from build123d import *

# Parameters (mm, degrees)
SKETCH2_W           = 96
SKETCH2_H           = 48
BOSS_EXTRUDE1_DEPTH = 12.7
SKETCH1_R           = 48
SKETCH1_R_2         = 23.5
SKETCH1_R_3         = 1
BOSS_EXTRUDE2_DEPTH = 12.7
SKETCH1_2_R         = 23.5
SKETCH1_2_R_2       = 1
CUT_EXTRUDE1_DEPTH  = 12.7
SKETCH3_R           = 30
CUT_EXTRUDE3_DEPTH  = 5
CHAMFER1_SIZE       = 0.5


with BuildPart() as part:
    # Sketch2 → Boss-Extrude1 (new body)
    with BuildSketch(Plane(origin=(0, 0, 0), x_dir=(1, 0, 0), z_dir=(0, 1, 0))):
        with Locations((0, 24)):
            Rectangle(SKETCH2_W, SKETCH2_H)
    extrude(amount=BOSS_EXTRUDE1_DEPTH)

    # Sketch1 → Boss-Extrude2 (add)
    with BuildSketch(Plane(origin=(0, 0, 0), x_dir=(1, 0, 0), z_dir=(0, 1, 0))):
        Circle(SKETCH1_R)
        Circle(SKETCH1_R_2, mode=Mode.SUBTRACT)
        with Locations((0, 44)):
            Circle(SKETCH1_R_3, mode=Mode.SUBTRACT)
        with Locations((34.400585229, 27.433551282)):
            Circle(SKETCH1_R_3, mode=Mode.SUBTRACT)
        with Locations(Location((42.896828136, -9.790921094, 0), (0, 0, 270))):
            Circle(SKETCH1_R_3, mode=Mode.SUBTRACT)
        with Locations(Location((19.090884521, -39.642630188, 0), (0, 0, 270))):
            Circle(SKETCH1_R_3, mode=Mode.SUBTRACT)
        with Locations(Location((-19.090884521, -39.642630188, 0), (0, 0, 270))):
            Circle(SKETCH1_R_3, mode=Mode.SUBTRACT)
        with Locations(Location((-42.896828136, -9.790921094, 0), (0, 0, 270))):
            Circle(SKETCH1_R_3, mode=Mode.SUBTRACT)
        with Locations((-34.400585229, 27.433551282)):
            Circle(SKETCH1_R_3, mode=Mode.SUBTRACT)
    extrude(amount=BOSS_EXTRUDE2_DEPTH)

    # Sketch1_2 → Cut-Extrude1 (cut)
    with BuildSketch(Plane(origin=(0, 0, 0), x_dir=(1, 0, 0), z_dir=(0, 1, 0))):
        with Locations(Location((0, 0, 0), (0, 0, 270))):
            Circle(SKETCH1_2_R)
        with Locations(Location((0, 44, 0), (0, 0, 270))):
            Circle(SKETCH1_2_R_2)
        with Locations(Location((34.400585229, 27.433551282, 0), (0, 0, 270))):
            Circle(SKETCH1_2_R_2)
        with Locations(Location((-34.400585229, 27.433551282, 0), (0, 0, 270))):
            Circle(SKETCH1_2_R_2)
    extrude(amount=CUT_EXTRUDE1_DEPTH, mode=Mode.SUBTRACT)

    # Sketch3 → Cut-Extrude3 (cut)
    with BuildSketch(Plane(origin=(0, 0, 0), x_dir=(1, 0, 0), z_dir=(0, 1, 0))):
        with Locations(Location((0, 0, 0), (0, 0, 270))):
            Circle(SKETCH3_R)
    extrude(amount=CUT_EXTRUDE3_DEPTH, mode=Mode.SUBTRACT)

    # Chamfer1
    chamfer1_edges = [part.edges().sort_by_distance(p)[0] for p in [
        (0, 12.7, -48),
        (-48, 12.7, -24),
        (0, 12.7, 48),
        (-23.5, 12.7, 0),
        (48, 12.7, -24),
    ]]
    chamfer(chamfer1_edges, length=CHAMFER1_SIZE)


solid = part.part
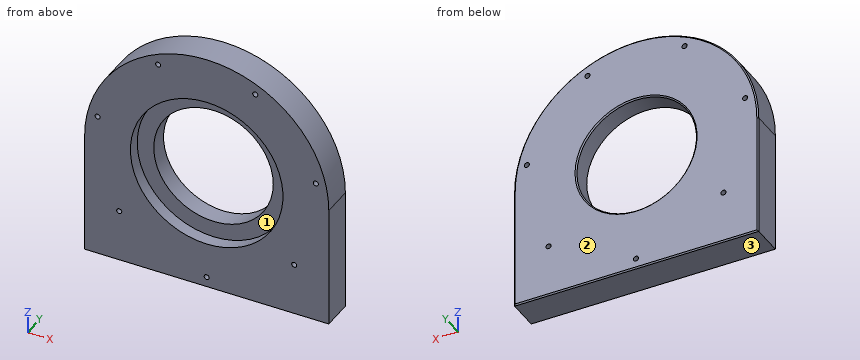
Can you work these out from the model? Positions are in its coordinate system, mm. Face numbers are marked on the shaded views. Round coordinates to 2 decimals unless told otherwise and drop trailing zeros. Write item = value, one per line. Start each with the question number.
(1) If I drill on probe 1 along Z at (x, y) = (15.5, 0.5); probe 2 along Z at (x, y) = (-15, 5.75); probe 3 along Z at (x, y) = (-19, 6.5), over which ranges is the centre line in solid material (lowest first)? Write a range as [from, to].
(2) For P1, Ø1.6, axis at x = 34.4, z = -27.43, coming from the +Y side; P2, Ø3, axis at y = 2, z = 11, coming from the +X side; P3, Ø5, axis at y = 10.5, z = 29, coming from the -X side; P4, Ø3, axis at y = 2, z = 12.5, coming from the +X side, each with a flat end and sliding along its axis, tell me the tip position at first contact or that it passes through.
(3) If we section it at A-A (y = 3.75): Give the number of separate pieces and of enclosed holes in the cut face, and give its area (3 significant figures).
(4) If we mould it in two halves opening along Z, with no side actions, what happens to the marked faces 1, 2 and 3? For each: released by +Z, released by -Z, zero draft, split by the parting line, or undercut.
Ans:
q1.probe_1 = [-48, -25.69], [25.69, 45.43]
q1.probe_2 = [-48, -18.09], [18.09, 45.6]
q1.probe_3 = [-48, -13.83], [13.83, 38.65], [40.64, 44.08]
q2.P1 = through
q2.P2 = 47.05
q2.P3 = -40.02
q2.P4 = 46.72
q3.separate_pieces = 1
q3.enclosed_holes = 8
q3.area = 5,380 mm²
q4.face_1 = undercut
q4.face_2 = zero draft
q4.face_3 = released by -Z
